Part model, mm, in its own coordinate system. A direction names the side the tool comes from. Coordinates: 2 decimals unless noted, no trailing zeros. Loops run counter-clockwise (first coordinate to the right, second up) from the corner with the lowest first, then second, coordinate; pieces in that order, holes last.
```python
from build123d import *

# Parameters (mm, degrees)
SKETCH1_W           = 38
SKETCH1_H           = 20
BOSS_EXTRUDE1_DEPTH = 2
BOSS_EXTRUDE2_DEPTH = 3
BOSS_EXTRUDE3_DEPTH = 2
SKETCH4_R           = 1.3
CUT_EXTRUDE1_DEPTH  = 51.865017448
CUT_EXTRUDE2_START  = -1
CUT_EXTRUDE2_DEPTH  = 2
SKETCH6_R           = 3.75
CUT_EXTRUDE3_DEPTH  = 2.4
SKETCH7_W           = 44
SKETCH7_H           = 6
CUT_EXTRUDE4_DEPTH  = 34.693471178
SKETCH8_R           = 2
BOSS_EXTRUDE4_DEPTH = 8
FILLET1_R           = 0.8
FILLET2_R           = 5
SKETCH9_R           = 1.5
CUT_EXTRUDE5_DEPTH  = 10


with BuildPart() as part:
    # Sketch1 → Boss-Extrude1 (new body)
    with BuildSketch(Plane.XY):
        Rectangle(SKETCH1_W, SKETCH1_H)
    extrude(amount=BOSS_EXTRUDE1_DEPTH)

    # Sketch2 → Boss-Extrude2 (add)
    with BuildSketch(Plane(origin=(19, 0, 0), x_dir=(0, 0, -1), z_dir=(1, 0, 0))):
        with BuildLine():
            Line((-2, 10), (0, 10))
            Line((0, 10), (19.347296355, 6.588549649))
            ThreePointArc((19.347296355, 6.588549649), (20.532088886, 5.904509362), (21, 4.618934143))
            Line((21, 4.618934143), (21, -4.618934143))
            ThreePointArc((21, -4.618934143), (20.532088886, -5.904509362), (19.347296355, -6.588549649))
            Line((19.347296355, -6.588549649), (0, -10))
            Line((0, -10), (-2, -10))
            Line((-2, -10), (-2, 10))
        make_face()
    boss_extrude2 = extrude(amount=BOSS_EXTRUDE2_DEPTH)

    # Mirror1: Boss-Extrude2 across plane
    add(boss_extrude2.mirror(Plane(origin=(0, 0, 0), x_dir=(0, 0, 1), z_dir=(1, 0, 0))))

    # Sketch3 → Boss-Extrude3 (add)
    with BuildSketch(Plane(origin=(0, 0, 0), x_dir=(-1, 0, 0), z_dir=(0, 0, -1))):
        Polygon((-22, -10), (-17.5, -14.5), (17.5, -14.5), (22, -10), align=None)
        Polygon((-22, 10), (22, 10), (17.5, 14.5), (-17.5, 14.5), align=None)
    extrude(amount=-BOSS_EXTRUDE3_DEPTH)

    # Sketch4 → Cut-Extrude1 (cut, through all)
    with BuildSketch(Plane.ZY.offset(22)):
        with Locations((-17, 0)):
            Circle(SKETCH4_R)
    extrude(amount=-CUT_EXTRUDE1_DEPTH, mode=Mode.SUBTRACT)

    # Sketch5 → Cut-Extrude2 (cut)
    with BuildSketch(Plane.ZY.offset(-19).offset(CUT_EXTRUDE2_START)):
        with BuildLine():
            Line((-0.5, -2.1), (-17, -3.9))
            ThreePointArc((-17, -3.9), (-20.9, 0), (-17, 3.9))
            Line((-17, 3.9), (-0.5, 2.1))
            ThreePointArc((-0.5, 2.1), (1.6, 0), (-0.5, -2.1))
        make_face()
    extrude(amount=-CUT_EXTRUDE2_DEPTH, mode=Mode.SUBTRACT)

    # Sketch6 → Cut-Extrude3 (cut)
    with BuildSketch(Plane.ZY.offset(-19)):
        with Locations((-17, 0)):
            Circle(SKETCH6_R)
    extrude(amount=-CUT_EXTRUDE3_DEPTH, mode=Mode.SUBTRACT)

    # Sketch7 → Cut-Extrude4 (cut, through all)
    with BuildSketch(Plane(origin=(0, 0, 0), x_dir=(-1, 0, 0), z_dir=(0, 0, -1))):
        with Locations((0, 13)):
            Rectangle(SKETCH7_W, SKETCH7_H)
    extrude(amount=-CUT_EXTRUDE4_DEPTH, mode=Mode.SUBTRACT)

    # Sketch8 → Boss-Extrude4 (add)
    with BuildSketch(Plane.ZY.offset(22)):
        with Locations((-17, 0)):
            Circle(SKETCH8_R)
    extrude(amount=-BOSS_EXTRUDE4_DEPTH)

    # Fillet1
    fillet1_edges = [part.edges().sort_by_distance(p)[0] for p in [
        (-19, 0, -19),
    ]]
    fillet(fillet1_edges, radius=FILLET1_R)

    # Fillet2
    fillet2_edges = [part.edges().sort_by_distance(p)[0] for p in [
        (-19, 0, 0),
        (19, 0, 0),
    ]]
    fillet(fillet2_edges, radius=FILLET2_R)

    # Sketch9 → Cut-Extrude5 (cut)
    with BuildSketch(Plane(origin=(0, 0, 0), x_dir=(-1, 0, 0), z_dir=(0, 0, -1))):
        with Locations((-10, 5)):
            Circle(SKETCH9_R)
        with Locations((9.5, -10.5)):
            Circle(SKETCH9_R)
    extrude(amount=-CUT_EXTRUDE5_DEPTH, mode=Mode.SUBTRACT)


solid = part.part
```
Q1. Probe line 1 (Y direction, x = 10, z = 1.3); line 2 (X direction, y = 8.25, z = -6.25); line 3 (Z direction, x = -4.5, y = -2). List the from-to ranges inside material, lowest first.
Q2. Saw through at C-C (z = -1). List the corners of the cut face in (x, y), plus the area to 3 significant figures.
Q3. Saw through at D-D (y = 0). List the corners of the cut face in (x, z).
Q4. Saw through at A-A (x = -9.5). List the corners of the cut face in (y, z).
Q5. Saw through at B-B (y = -10.5). List the corners of the cut face in (x, z).
Q6. Tool access for faces 1 (the flat face through (-14, 0, -17)), 2 (the flat face through (20.611, 8.318, -9.538)), 3 (the flat face through (20.986, -2.987, -8.635)), 4 (the flat face through (19, 0, -11)): list every direction of +Z, -Z, +X, -X, +Y, -Y with a clear straight run to the whole face (end or side of a thin tool).
Q7. Mould opens along Z. For faces 5 (the flat face through (19.8, 0.1, -21)), 6 (the flat face through (22, 5, -7)), 7 (the cylindrical face through (-16.1, -1.2, -18.6)), 8 (the cylindrical face through (21, 0, 1.6)) say: released by +Z, released by -Z, zero draft, split by the parting line, or undercut.
Q8. Drop flat-ended pins along their axis: P1, Ø4.5, axis at y = -0.5, z = -16, coming from the +X side; P2, Ø1, axis at x = -14, y = -4, coming from the -Z side; P3, Ø7.5, axis at x = -11, y = -1, coming from the -Z side. Give the stop position or say it passes through.
Checked values:
1. line 1: y = -14.5 to 3.5, 6.5 to 10
1. line 2: x = -22 to -19, 19 to 22
1. line 3: z = 0 to 2
2. outline: (-22, -9.82) - (-17, -9.82) - (-17, 9.82) - (-22, 9.82) - close; (17, -9.82) - (22, -9.82) - (22, -2.15) - (20, -2.15) - (20, 2.15) - (22, 2.15) - (22, 9.82) - (17, 9.82) - close
2. area: 188 mm2
3. outline: (-22, -21) - (-19, -21) - (-19, -19.8) arc R0.8 cw to (-18.2, -19) - (-14, -19) - (-14, -15) - (-18.2, -15) arc R0.8 cw to (-19, -14.2) - (-19, -5) arc R5 cw to (-14, 0) - (14, 0) arc R5 cw to (19, -5) - (19, -13.25) - (20, -13.25) - (20, 1.6) - (22, 1.6) - (22, 2) - (-22, 2) - close; (19, -21) - (22, -21) - (22, -20.9) - (20, -20.9) - (20, -20.75) - (19, -20.75) - close
4. outline: (-14.5, 0) - (-12, 0) - (-12, 2) - (-14.5, 2) - close; (-9, 0) - (10, 0) - (10, 2) - (-9, 2) - close
5. outline: (-21.5, 0) - (-11, 0) - (-11, 2) - (-21.5, 2) - close; (-8, 0) - (21.5, 0) - (21.5, 2) - (-8, 2) - close
6. face 1: -Z, +X, +Y, -Y
6. face 2: -Z, +X, -X, +Y
6. face 3: +X
6. face 4: -Z, +Y, -Y
7. face 5: released by -Z
7. face 6: zero draft
7. face 7: undercut
7. face 8: undercut
8. P1: stops at x = -14
8. P2: stops at z = -0.03
8. P3: stops at z = -19
